Autodesk Inventor part; units mm, degrees
ref_plane "YZ Plane" through (0, 0, 0) normal (1, 0, 0) x (0, 1, 0)
ref_plane "XZ Plane" through (0, 0, 0) normal (0, 1, 0) x (-1, 0, 0)
ref_plane "XY Plane" through (0, 0, 0) normal (0, 0, 1) x (1, 0, 0)
sketch "Sketch9" plane through (0, 0, 0) normal (0, 1, 0) x (-1, 0, 0)
  line L0 (15, 15) -> (-15, 15)
  line L1 (-15, 15) -> (-15, -15)
  line L2 (-15, -15) -> (15, -15)
  line L3 (15, -15) -> (15, 15)
  line L4 (15, 15) -> (-15, -15) construction
  line L5 (-15, 15) -> (15, -15) construction
  line L6 (-13, 13) -> (13, 13)
  line L7 (13, 13) -> (13, -13)
  line L8 (13, -13) -> (-13, -13)
  line L9 (-13, -13) -> (-13, 13)
  point P0 (0, 0)
  dimension "d172" = 30
  dimension "d173" = 30
  dimension "d174" = 2
extrude "Extrusion3" add sketch "Sketch9" against normal blind 320
sketch "Sketch10" plane through (0, 0, 0) normal (1, 0, 0) x (0, 1, 0)
  line L0 (0, 15) -> (0, -15) construction
  line L1 (0, 15) -> (-320, 15) construction
  line L2 (-320, -15) -> (-320, 15) construction
  line L3 (0, -15) -> (-320, -15) construction
  line L4 (-148.5, 8.5) -> (-131.5, 8.5)
  line L5 (-131.5, 8.5) -> (-131.5, -8.5)
  line L6 (-131.5, -8.5) -> (-148.5, -8.5)
  line L7 (-148.5, -8.5) -> (-148.5, 8.5)
  line L8 (-148.5, 8.5) -> (-131.5, -8.5) construction
  line L9 (-131.5, 8.5) -> (-148.5, -8.5) construction
  line L10 (-308.5, 8.5) -> (-291.5, 8.5)
  line L11 (-291.5, 8.5) -> (-291.5, -8.5)
  line L12 (-291.5, -8.5) -> (-308.5, -8.5)
  line L13 (-308.5, -8.5) -> (-308.5, 8.5)
  line L14 (-308.5, 8.5) -> (-291.5, -8.5) construction
  line L15 (-291.5, 8.5) -> (-308.5, -8.5) construction
  line L16 (-428.5, 8.5) -> (-411.5, 8.5)
  line L17 (-411.5, 8.5) -> (-411.5, -8.5)
  line L18 (-411.5, -8.5) -> (-428.5, -8.5)
  line L19 (-428.5, -8.5) -> (-428.5, 8.5)
  line L20 (-428.5, 8.5) -> (-411.5, -8.5) construction
  line L21 (-411.5, 8.5) -> (-428.5, -8.5) construction
  circle A0 centre (-470, 0) radius 8.5
  line L22 (0, 0) -> (30, 0)
  circle A1 centre (-140, 0) radius 8.5
  circle A2 centre (-300, 0) radius 8.5
  circle A3 centre (-420, 0) radius 8.5
  dimension "d177" = 17
  dimension "d178" = 17
  dimension "d181" = 30
  dimension "d182" = 170
  dimension "d183" = 330
  dimension "d184" = 450
  dimension "d185" = 500
  dimension "d186" = 17
extrude "Extrusion4" cut sketch "Sketch10" along normal through all contours A1 | A2
properties part number "PNS 756 FDS 1200 way tube 3_1600" material "Stainless Steel"
Verification items for the finished model (mm, model axes). A direction names the side the tool comes from. Give positions to 0.01 mm unless a question says otherwise; leave off trailing zeros. Order: outer loops, then holes, each group sorted by start corner. A loop starts at its lowest first (then second) coordinate and runs counter-clockwise, first axis right, second up. Notation, with made-up numbers: (-8.5, -39.5) - (14.5, -39.5) arc R19 cw to (14.5, -9.5) - close; hole circle Ø1 at (51, 16). An arc over 180 degrees is marked (long way). Answer as CSV lines item,"result". Start each with the question number.
Item 1: Section check A-A, the plane z = 0. Record the boundary of the cut face in (x, y), plus the area to 3 significant figures.
Item 2: Mould release check, pull along X, two halves, no side actions. Record for faces 1 (the face through (13.99, -131.89, -2.55)), 2 (the face through (0, -158, 13)), 3 (the face through (-15, -158, 0)): released by +X, released by -X, zero draft, split by the parting line, or undercut.
Item 3: Material ranges on L1, parallel to Y at x = 14.15, z = 0; L2, parallel to X at y = -170, z = 0.75, recorded low to high.
Item 4: Section check C-C, the plane y = -201.5. Record the boundary of the cut face in (x, z), plus the area to 3 significant figures.
Item 5: Section check D-D, the plane y = -140. Record the boundary of the cut face in (x, z).
Item 6: Gauge pin test, flat end, axial feed: pin 1 (13.5 mm diameter, centred on y = -140, z = 0, fed in from +X). Record the tip position at first contact, or that the pin passes through.
Item 7: Section check B-B, the plane x = 0.75. Record the boundary of the cut face in (y, z), plus the area to 3 significant figures.
Item 8: Access from +Z, -Z, +X, -X, +Y, -Y to the whole of each face (thin tool, end or side, straight path). Record for faces 4 (the face through (13.99, -308.49, -0.37)), 5 (the face through (0, -158, -13)), 6 (the face through (0, -158, -15)).
Filled in:
1,outline,"(-15, -320) - (-13, -320) - (-13, 0) - (-15, 0) - close; (13, -320) - (15, -320) - (15, -308.5) - (13, -308.5) - close; (13, -291.5) - (15, -291.5) - (15, -148.5) - (13, -148.5) - close; (13, -131.5) - (15, -131.5) - (15, 0) - (13, 0) - close"
1,area,"1,210 mm^2"
2,face 1,"zero draft"
2,face 2,"undercut"
2,face 3,"released by -X"
3,L1,"-320 to -308.5, -291.5 to -148.5, -131.5 to 0"
3,L2,"-15 to -13, 13 to 15"
4,outline,"(-15, -15) - (15, -15) - (15, 15) - (-15, 15) - close; hole (-13, -13) - (13, -13) - (13, 13) - (-13, 13) - close"
4,area,"224 mm^2"
5,outline,"(-15, -15) - (15, -15) - (15, -8.5) - (13, -8.5) - (13, -13) - (-13, -13) - (-13, 13) - (13, 13) - (13, 8.5) - (15, 8.5) - (15, 15) - (-15, 15) - close"
6,pin 1,"x = -13"
7,outline,"(-320, -15) - (0, -15) - (0, -13) - (-320, -13) - close; (-320, 13) - (0, 13) - (0, 15) - (-320, 15) - close"
7,area,"1,280 mm^2"
8,face 4,"+X"
8,face 5,"+Y, -Y"
8,face 6,"-Z, +X, -X, +Y, -Y"
